CAD build for the part. Positions are in the model's coordinates, mm. Face numbers are marked on the shaded views. A direction names the side the tool comes from. Coordinates: 2 decimals unless noted, no trailing zeros. Order: outer loops, then holes, each group sorted by start corner. A loop starts at its lowest first (then second) coordinate and runs counter-clockwise, first axis right, second up.
from build123d import *

# Parameters (mm, degrees)
F1_DEPTH = 25
F2_R     = 1.4
F3_DEPTH = 6
F4_R     = 0.5


with BuildPart() as f1:
    # F0 (on Front) → F1 (new body)
    with BuildSketch(Plane.XZ):
        with BuildLine():
            Line((0, 1.9), (0, 0))
            Line((0, 0), (20.1, 0))
            Line((20.1, 0), (20.1, 1.9))
            ThreePointArc((20.1, 1.9), (19.35, 2.65), (20.1, 3.4))
            Line((20.1, 3.4), (20.1, 5.3))
            Line((20.1, 5.3), (0, 5.3))
            Line((0, 5.3), (0, 3.4))
            ThreePointArc((0, 3.4), (0.75, 2.65), (0, 1.9))
        make_face()
    extrude(amount=F1_DEPTH)

    # F2 (on face) → F3 (join)
    with BuildSketch(Plane.XZ.offset(25)):
        with Locations((4.2, 2.65)):
            Circle(F2_R)
        with Locations((15.9, 2.65)):
            Circle(F2_R)
    extrude(amount=F3_DEPTH)

    # F4
    f4_edges = [f1.edges().sort_by_distance(p)[0] for p in [
        (20.1, -12.5, 5.3),
        (20.1, -12.5, 3.4),
        (20.1, -12.5, 1.9),
        (20.1, -12.5, 0),
        (0, -12.5, 5.3),
        (0, -12.5, 0),
        (0, -12.5, 1.9),
        (0, -12.5, 3.4),
    ]]
    fillet(f4_edges, radius=F4_R)


solid = f1.part
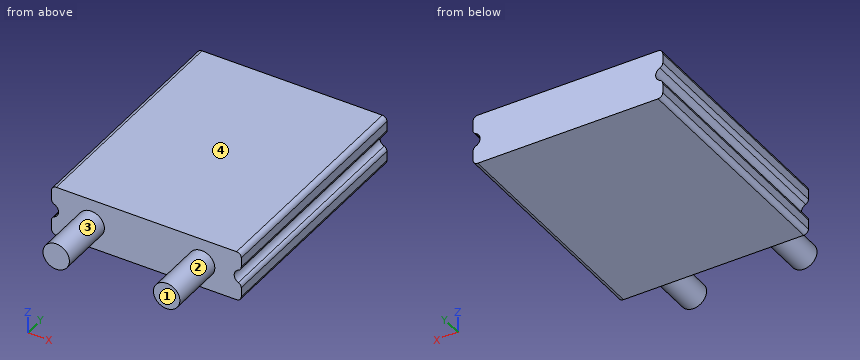
1) Slice it at C-C (z = 2.65). List the corners of the cut face in (x, y).
2) Which spindle directions (+Z, -Z, +X, -X, +Y, -Y) get a long thin tool onto all of the face, cutting with end or side? Do the marked faces 3 and 4. Say none if no direction does.
3) Drill centre lines: probe 1 along Y at (x, z) = (1.25, 4.8); probe 2 along X at (y, z) = (-25.5, 3.1); probe 3 along X at (y, z) = (-22.5, 2.45). Where is each one in solid material? Low to high.
4) Slice it at D-D (y = -29). List the corners of the cut face in (x, z), plus the area to 3 significant figures.
5) Slice it at B-B (y = -15.5). List the corners of the cut face in (x, z).
6) Two-plate mould, pull along X, no slides. Class the marked faces 1 and 2: released by +X, released by -X, zero draft, split by the parting line, or undercut.
7) Slice it at A-A (x = 4.2). List the corners of the cut face in (y, z), plus the area to 3 significant figures.
Worked out:
1. outline: (0.75, -25) - (2.8, -25) - (2.8, -31) - (5.6, -31) - (5.6, -25) - (14.5, -25) - (14.5, -31) - (17.3, -31) - (17.3, -25) - (19.35, -25) - (19.35, 0) - (0.75, 0) - close
2. face 3: -Y
2. face 4: +Z, +X, -X, +Y, -Y
3. probe 1: y = -25 to 0
3. probe 2: x = 2.87 to 5.53, 14.57 to 17.23
3. probe 3: x = 0.72 to 19.38
4. outline: circle Ø2.8 at (4.2, 2.65); circle Ø2.8 at (15.9, 2.65)
4. area: 12.3 mm2
5. outline: (0, 0.5) arc R0.5 ccw to (0.5, 0) - (19.6, 0) arc R0.5 ccw to (20.1, 0.5) - (20.1, 1.5) arc R0.5 ccw to (19.8, 1.96) arc R0.75 cw to (19.8, 3.34) arc R0.5 ccw to (20.1, 3.8) - (20.1, 4.8) arc R0.5 ccw to (19.6, 5.3) - (0.5, 5.3) arc R0.5 ccw to (0, 4.8) - (0, 3.8) arc R0.5 ccw to (0.3, 3.34) arc R0.75 cw to (0.3, 1.96) arc R0.5 ccw to (0, 1.5) - close
6. face 1: zero draft
6. face 2: undercut
7. outline: (-31, 1.25) - (-25, 1.25) - (-25, 0) - (0, 0) - (0, 5.3) - (-25, 5.3) - (-25, 4.05) - (-31, 4.05) - close
7. area: 149 mm2
